Input: part model. Units: mm. Frame: model coordinates. Face numbers are marked on the shaded views. A direction names the side the tool comes from. Give positions to 0.01 mm unless a question says otherwise; leave off trailing zeros. Loops run counter-clockwise (first coordinate to the right, second up) from the corner with the lowest first, then second, coordinate; pieces in that order, holes last. Notation, with made-up numbers: (69, 36.5) -> (99, 36.5) arc R14 cw to (99, 51.5) -> close; hole circle Ø5 at (15.25, -10.75). An arc over 180 degrees is marked (long way). Use CSV: the item, a comma, the result in double quotes.
```python
from build123d import *

# Parameters (mm, degrees)
ESQUISSE2_W             = 20
ESQUISSE2_H             = 2
ESQUISSE2_W_2           = 16.5
ESQUISSE2_H_2           = 16.5
BOSS_EXTRU_1_DEPTH      = 5
ENL_V_MAT_EXTRU_1_DEPTH = 17
ENL_V_MAT_EXTRU_2_DEPTH = 17


with BuildPart() as part:
    # Esquisse2 → Boss.-Extru.1 (new body)
    with BuildSketch(Plane(origin=(0, 0, 0), x_dir=(1, 0, 0), z_dir=(0, 1, 0))):
        with Locations((10, 1)):
            Rectangle(ESQUISSE2_W, ESQUISSE2_H)
        with Locations((-8.25, 1)):
            Rectangle(ESQUISSE2_W_2, ESQUISSE2_H_2)
    extrude(amount=BOSS_EXTRU_1_DEPTH)

    # Esquisse3 → Enlèv. mat.-Extru.1 (cut)
    with BuildSketch(Plane(origin=(0, 0, -9.25), x_dir=(-1, 0, 0), z_dir=(0, 0, -1))):
        with BuildLine():
            Line((0, 5), (0, 3.654066972))
            add(Edge.make_bspline(
                [(0, 3.654066972), (8.276287375, 2.347006327), (16.5, 0.744396355)],
                knots=[0, 0, 0, 1, 1, 1], degree=2))
            Line((16.5, 0.744396355), (18.688542218, 4.20494166))
            Line((18.688542218, 4.20494166), (16.723031274, 6.238601979))
            Line((16.723031274, 6.238601979), (3.598874135, 6.46224909))
            Line((3.598874135, 6.46224909), (0, 5))
        make_face()
    extrude(amount=-ENL_V_MAT_EXTRU_1_DEPTH, mode=Mode.SUBTRACT)

    # Esquisse4 → Enlèv. mat.-Extru.2 (cut)
    with BuildSketch(Plane.XY):
        with BuildLine():
            Line((0, 3.654066972), (0, 5))
            Line((0, 5), (7.983599521, 5))
            add(Edge.make_bspline(
                [(0, 3.654066972), (3.907893525, 4.793033974), (7.983599521, 5)],
                knots=[0, 0, 0, 1, 1, 1], degree=2))
        make_face()
    extrude(amount=-ENL_V_MAT_EXTRU_2_DEPTH, mode=Mode.SUBTRACT)


solid = part.part
```
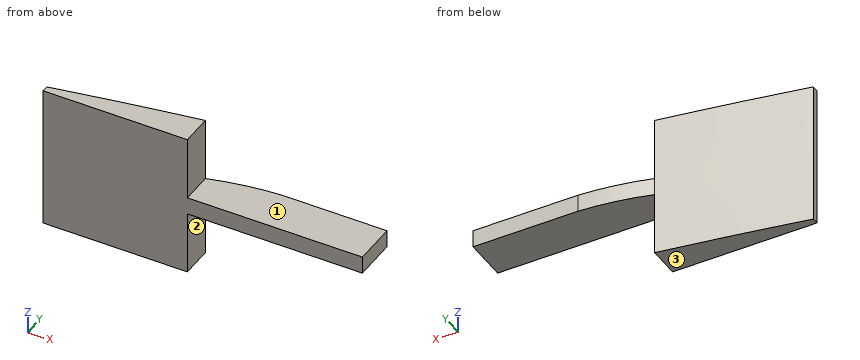
1) Contact query for flat-ended pins moving along their axis: pin 1 (1.5 mm diameter, centred on x = 1, y = 2, fed in from +Z); pin 2 (1.1 mm diameter, centred on y = 1, z = -6.5, fed in from +X); pin 3 (3 mm diameter, centred on x = 6.5, y = 3, fed in from -Z). Output: stop coordinate, or through.
From the geometry:
pin 1,"stops at z = 0"
pin 2,"stops at x = 0"
pin 3,"stops at z = -2"
2) Section query A-A (x = 16.5). Return loops of the section in (y, z), then the cut area to 3 significant figures.
From the geometry:
outline,"(0, -2) -> (5, -2) -> (5, 0) -> (0, 0) -> close"
area,"10.0 mm^2"
3) Reachability of the marked faces 1, 2 and 3 from +Z, -Z, +X, -X, +Y, -Y: full face, straight path, thin tool, end or side. Return the list, or none.
From the geometry:
face 1,"+Z, +X, +Y, -Y"
face 2,"-Z, +X, +Y, -Y"
face 3,"-Z, +X, -X, +Y, -Y"
4) Ray query, line 1 (Z direction, x = 16, y = 1.75); line 2 (X direction, y = 0.55, z = 2.5); line 3 (Y direction, x = -6.5, z = 3). Return the intervals inside material, ascending.
From the geometry:
line 1,"z = -2 to 0"
line 2,"x = -16.5 to 0"
line 3,"y = 0 to 2.58"
